Could you check a few things on this drawing? It's one solid part, dimensions in mm from its lowest x, y, z. A direction names the side the tool comes from. Coordinates: 2 decimals unless noted, no trailing zeros. Order: outer loops, then holes, each group sorted by start corner. A loop starts at its lowest first (then second) coordinate and runs counter-clockwise, first axis right, second up.
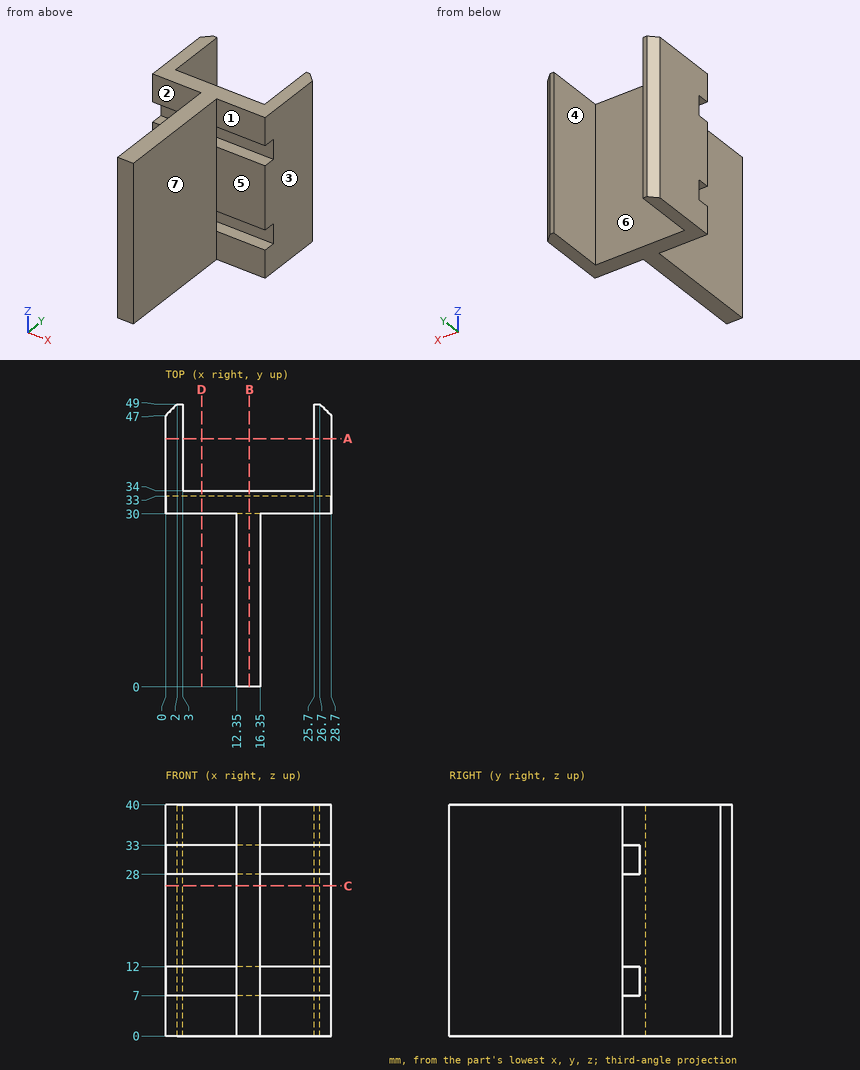
1. Imagine slicing it at C-C on z = 26. Please give me the cut outline in (x, y).
Completed:
outline: (0, 30) - (12.35, 30) - (12.35, 0) - (16.35, 0) - (16.35, 30) - (28.7, 30) - (28.7, 47) - (26.7, 49) - (25.7, 49) - (25.7, 34) - (3, 34) - (3, 49) - (2, 49) - (0, 47) - close
2. Thinking about a two-plate mould opening in X: for the marked faces 5, 6 and 7, which applies, pulls with the +X half, pulls with the -X half, needs draft (parallel to the pull), parting line crosses it, or undercut?
Completed:
face 5: needs draft
face 6: undercut
face 7: pulls with the +X half
3. Please list where these lines run through material, in increasing order: probe 1 along Z at (x, y) = (8.5, 30.5); probe 2 along X at (y, z) = (44, 21.5); probe 3 along Y at (x, z) = (14.5, 14).
Completed:
probe 1: z = 0 to 7, 12 to 28, 33 to 40
probe 2: x = 0 to 3, 25.7 to 28.7
probe 3: y = 0 to 34
4. On a 3-axis mill with a long thin cutter (end or side, diameter ignored), from which of +Z, -Z, +X, -X, +Y, -Y can I reach the whole of each face in a straight line? I mean the marked faces 1, 2, 3 and 4. Say none if no direction works.
Completed:
face 1: +Z, -Z, +X, -Y
face 2: +Z, -Z, -X, -Y
face 3: +Z, -Z, +X, +Y, -Y
face 4: +Z, -Z, +Y
5. Imagine slicing it at B-B on x = 14.5. Please give me the cut outline in (y, z), then the cut area to 3 significant figures.
Completed:
outline: (0, 0) - (34, 0) - (34, 40) - (0, 40) - close; hole (30, 7) - (33, 7) - (33, 12) - (30, 12) - close; hole (30, 28) - (33, 28) - (33, 33) - (30, 33) - close
area: 1,330 mm2
6. Imagine slicing it at D-D on x = 6.25. Please give me the cut outline in (y, z), then the cut area to 3 significant figures.
Completed:
outline: (30, 0) - (34, 0) - (34, 40) - (30, 40) - (30, 33) - (33, 33) - (33, 28) - (30, 28) - (30, 12) - (33, 12) - (33, 7) - (30, 7) - close
area: 130 mm2
7. Imagine slicing it at A-A on y = 43. Please give me the cut outline in (x, z), then the cut area to 3 significant figures.
Completed:
outline: (0, 0) - (3, 0) - (3, 40) - (0, 40) - close; (25.7, 0) - (28.7, 0) - (28.7, 40) - (25.7, 40) - close
area: 240 mm2
8. I'm going to push flat-ended pins straight in: pin 1 (12 mm diameter, centred on y = 21, z = 27, fed in from +X); pin 2 (2 mm diameter, centred on x = 14, z = 9, fed in from +Y); pin 3 (6 mm diameter, centred on x = 25, z = 17, fed in from -Y). Where does each tip first touch, or does it pass through?
Completed:
pin 1: stops at x = 16.35
pin 2: stops at y = 34
pin 3: stops at y = 30
